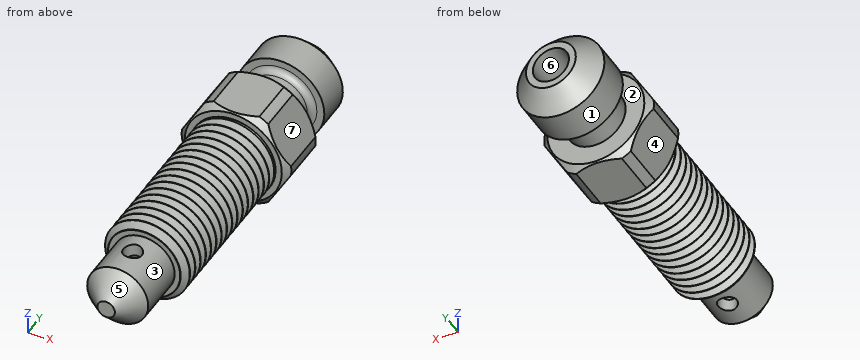
```python
from build123d import *

# Parameters (mm, degrees)
CHAMFER1_SIZE           = 0.5
FILLET1_R               = 0.5
CUT_EXTRUDE1_DEPTH      = 32.373276845
CUT_EXTRUDE1_DEPTH_BACK = 32.373276845
SKETCH2_R               = 0.75
SKETCH3_OUTSIDE_W       = 17.434
SKETCH3_OUTSIDE_H       = 17.434
CUT_EXTRUDE2_DEPTH      = 5
CHAMFER2_SIZE           = 0.5


with BuildPart() as part:
    # Sketch1 → Revolve1 (revolve)
    with BuildSketch(Plane.XY, mode=Mode.PRIVATE) as revolve1_sk:
        Polygon((0, 0), (-0.7, 0), (-2.45, 1.75), (-2.45, 5.75), (-3.4, 5.75), (-3.4, 19.25), (-4.4, 19.25), (-4.4, 23.95), (-2.4, 23.95), (-2.4, 26.45), (-3.5, 26.45), (-3.5, 29.25), (-2, 30.75), (-1.45, 30.75), (-1.45, 2), (0, 2), align=None)
    revolve(revolve1_sk.sketch.rotate(Axis((0, 1.982963205, 0), (0, 1, 0)), 270), axis=Axis((0, 1.982963205, 0), (0, 1, 0)))

    # Chamfer1
    chamfer1_edges = [part.edges().sort_by_distance(p)[0] for p in [
        (0, 23.95, 4.4),
        (0, 19.25, 4.4),
    ]]
    chamfer(chamfer1_edges, length=CHAMFER1_SIZE)

    # Fillet1
    fillet1_edges = [part.edges().sort_by_distance(p)[0] for p in [
        (0, 26.45, 2.4),
    ]]
    fillet(fillet1_edges, radius=FILLET1_R)

    # Sketch2 → Cut-Extrude1 (cut, two sides: drawn at the far end of the back side and taken through both)
    with BuildSketch(Plane.XY.offset(-CUT_EXTRUDE1_DEPTH_BACK)):
        with Locations((0, 4)):
            Circle(SKETCH2_R)
    extrude(amount=CUT_EXTRUDE1_DEPTH + CUT_EXTRUDE1_DEPTH_BACK, mode=Mode.SUBTRACT)

    # Sketch3 outside → Cut-Extrude2 (cut)
    with BuildSketch(Plane(origin=(0, 23.95, 0), x_dir=(1, 0, 0), z_dir=(0, 1, 0))):
        Rectangle(SKETCH3_OUTSIDE_W, SKETCH3_OUTSIDE_H)
        Polygon((4.618802154, 0), (2.309401077, 4), (-2.309401077, 4), (-4.618802154, 0), (-2.309401077, -4), (2.309401077, -4), align=None, mode=Mode.SUBTRACT)
    extrude(amount=-CUT_EXTRUDE2_DEPTH, mode=Mode.SUBTRACT)

    # Chamfer2
    chamfer2_edges = [part.edges().sort_by_distance(p)[0] for p in [
        (0, 5.75, 3.4),
    ]]
    chamfer(chamfer2_edges, length=CHAMFER2_SIZE)

    # Sketch4 → Cut-Revolve1 (revolve, cut)
    with BuildSketch(Plane.XY, mode=Mode.PRIVATE) as cut_revolve1_sk:
        Polygon((3.4, 5.5), (3.4, 6.25), (2.750480947, 5.875), align=None)
        Polygon((3.4, 7.05), (2.750480947, 6.675), (3.4, 6.3), align=None)
        Polygon((3.4, 7.85), (2.750480947, 7.475), (3.4, 7.1), align=None)
        Polygon((3.4, 8.65), (2.750480947, 8.275), (3.4, 7.9), align=None)
        Polygon((3.4, 9.45), (2.750480947, 9.075), (3.4, 8.7), align=None)
        Polygon((3.4, 10.25), (2.750480947, 9.875), (3.4, 9.5), align=None)
        Polygon((3.4, 11.05), (2.750480947, 10.675), (3.4, 10.3), align=None)
        Polygon((3.4, 11.85), (2.750480947, 11.475), (3.4, 11.1), align=None)
        Polygon((3.4, 12.65), (2.750480947, 12.275), (3.4, 11.9), align=None)
        Polygon((3.4, 13.45), (2.750480947, 13.075), (3.4, 12.7), align=None)
        Polygon((3.4, 14.25), (2.750480947, 13.875), (3.4, 13.5), align=None)
        Polygon((3.4, 15.05), (2.750480947, 14.675), (3.4, 14.3), align=None)
        Polygon((3.4, 15.85), (2.750480947, 15.475), (3.4, 15.1), align=None)
        Polygon((3.4, 16.65), (2.750480947, 16.275), (3.4, 15.9), align=None)
        Polygon((3.4, 17.45), (2.750480947, 17.075), (3.4, 16.7), align=None)
        Polygon((3.4, 18.25), (2.750480947, 17.875), (3.4, 17.5), align=None)
        Polygon((3.4, 19.05), (2.750480947, 18.675), (3.4, 18.3), align=None)
    revolve(cut_revolve1_sk.sketch.rotate(Axis((0, 0, 0), (0, 1, 0)), 90), axis=Axis((0, 0, 0), (0, 1, 0)), mode=Mode.SUBTRACT)


solid = part.part
```
Read the model definition and answer for the solid it produces. Units are mm, in the model's axes. Face numbers are marked on the shaded views. A direction names the side the tool comes from. Coordinates: 2 decimals unless noted, no trailing zeros. Loops run counter-clockwise (first coordinate to the right, second up) from the corner with the lowest first, then second, coordinate; pieces in that order, holes last. Notation, with made-up numbers: (58.5, 39) - (79.5, 39) arc R32 cw to (79.5, 70) - close; hole circle Ø11 at (6.5, 18). An arc over 180 degrees is marked (long way). Answer in a Markdown table with one row per item.
1. Determine the mould class of the marked faces 4, 5, 6 and 7 for opening direction X: +X half, -X half, draft (parallel to the pull), parting line (faces both ways), or undercut.
Conclusion:
| item | result |
|---|---|
| face 4 | -X half |
| face 5 | parting line |
| face 6 | undercut |
| face 7 | +X half |
2. Which of the six approach directions +Z, -Z, +X, -X, +Y, -Y give full straight-line access (tool end or side, diameter ignored) to the marked faces 1, 2 and 3?
Conclusion:
| item | result |
|---|---|
| face 1 | +Y |
| face 2 | none |
| face 3 | -Y |
3. Given pin 1 (3.5 mm diameter, centred on x = 1, z = -0.5, fed in from -Y); pin 2 (1.4 mm diameter, centred on x = 0.5, z = 0, fed in from +Y); pin 3 (1.5 mm diameter, centred on y = 14, z = -3, fed in from -X); pin 4 (4 mm diameter, centred on y = 15, z = 3, fed in from -X), each flat-ended and moving along its own axis, determine where each tip first touches the part or whether it passes through.
Conclusion:
| item | result |
|---|---|
| pin 1 | stops at y = 0 |
| pin 2 | stops at y = 2 |
| pin 3 | stops at x = -2.51 |
| pin 4 | stops at x = -3.25 |
4. Straight lines are drawn through the part: line 1 (X direction, y = 4, z = -2.05); line 2 (X direction, y = 11.5, z = -0.5); line 3 (Y direction, x = -0.5, z = 2.5). For each, find the intervals that lie inside material, in ascending order.
Conclusion:
| item | result |
|---|---|
| line 1 | x = -1.34 to -0.75, 0.75 to 1.34 |
| line 2 | x = -2.75 to -1.36, 1.36 to 2.75 |
| line 3 | y = 5.75 to 23.95, 26.31 to 30.2 |
5. Find section A-A, the plane y = 4. Write down the section's boundary in (x, z), then the cut area to 3 significant figures.
Conclusion:
| item | result |
|---|---|
| outline | (-0.75, -2.33) - (-0.75, -1.24) arc R1.45 cw to (-0.75, 1.24) - (-0.75, 2.33) arc R2.45 ccw to start; (0.75, -2.33) arc R2.45 ccw to (0.75, 2.33) - (0.75, 1.24) arc R1.45 cw to (0.75, -1.24) - close |
| area | 9.17 mm² |
6. Find section B-B, the plane x = 0. Count the separate pieces of the cut face and the enclosed holes in it, then the cut area to 3 significant figures.
Conclusion:
| item | result |
|---|---|
| separate pieces | 3 |
| enclosed holes | 0 |
| area | 99.9 mm² |
